Autodesk Inventor part; units mm, degrees
ref_plane "YZ Plane" through (0, 0, 0) normal (1, 0, 0) x (0, 1, 0)
ref_plane "XZ Plane" through (0, 0, 0) normal (0, 1, 0) x (-1, 0, 0)
ref_plane "XY Plane" through (0, 0, 0) normal (0, 0, 1) x (1, 0, 0)
sketch "Sketch1" plane through (0, 0, 0) normal (0, 0, 1) x (1, 0, 0)
  line L0 (-35, 35) -> (35, 35)
  line L1 (35, 35) -> (35, -35)
  line L2 (35, -35) -> (-35, -35)
  line L3 (-35, -35) -> (-35, 35)
  circle A0 centre (0, 0) radius 20
  point P0 (35, 0)
  point P1 (0, 35)
  dimension "d0" = 70
  dimension "d1" = 40
extrude "Extrusion1" add sketch "Sketch1" along normal blind 6
chamfer "Chamfer1" distance 12 angle 45 4 edges at (35, 35, 3) (35, -35, 3) (-35, -35, 3) (-35, 35, 3)
fillet "Fillet1" radius 2 8 edges at (-23, 35, 3) (23, 35, 3) (35, 23, 3) (35, -23, 3) (23, -35, 3) (-23, -35, 3) (-35, -23, 3) (-35, 23, 3)
sketch "Sketch2" plane through (0, 0, 6) normal (0, 0, 1) x (1, 0, 0)
  circle A0 centre (0, 0) radius 32 construction
  point P0 (32, 0)
  dimension "d8" = 64
hole "Hole1" at (32, 0, 6) direction (0, 0, -1) diameter 5.1 end through all
pattern_circular "Circular Pattern1" count 4 over 360 about axis through (0, 0, -10) along (0, 0, 1) of "Hole1"
sketch "Sketch3" plane through (0, 0, 6) normal (0, 0, 1) x (1, 0, 0)
  circle A0 centre (0, 0) radius 23.75 construction
  point P0 (23.75, 0)
  dimension "d19" = 47.5
hole "Hole2" at (23.75, 0, 6) direction (0, 0, -1) diameter 3.2 end through all
pattern_circular "Circular Pattern2" count 4 over 360 about axis through (0, 0, -10) along (0, 0, 1) of "Hole2"
properties part number "plasma-box-spacer-6mm" material "Copper"
Verification items for the finished model (mm, model axes). Give positions to 0.01 mm unless a question says otherwise; leave off trailing zeros. Order: outer loops, then holes, each group sorted by start corner. A loop starts at its lowest first (then second) coordinate and runs counter-clockwise, first axis right, second up. Notation, with made-up numbers: M 29.5,40.25 L 84.5,40.25 A11 cw 84.5,44.25 Z; hole C -12,-17 d7. An arc over 180 degrees is marked long. Use one line per item in the form item = value. Start each with the question number.
Q1. Section check B-B (y = 0). Enter the section's corners in (x, z), then the cut area to 3 significant figures.
Q2. Scan lines: line 1 along Y through (x, z) = (0, 1.7); line 2 along Y through (x, z) = (-2, 2.25); line 3 along Y through (x, z) = (-30.5, 4.65). Record each from-to range of solid material in increasing order. Write a range as [from, to].
Q3. Section check A-A (x = 32). Enter the section's corners in (y, z), then the cut area to 3 significant figures.
Q4. Go/stop test with a flat-tipped pin: pin 1 Ø1.9 at (x, y) = (-23.75, 0) entering from +Z. Record where the tip stops, or that it passes through.
Q5. Section check C-C (z = 4.4). Count the separate pieces of the cut face and the enclosed holes in it, then the cut area to 3 significant figures.
Q6. Mould release check, pull along X, two halves, no side actions. Record for faces 1 (the flat face through (29, 29, 3)), 2 (the flat face through (15, 16, 0)), 3 (the cylindrical face through (-22.164, -0.208, 2.958)): +X half, -X half, draft (parallel to the pull), parting line (faces both ways), or undercut.
Evaluation:
q1.outline = M -35,0 L -34.55,0 L -34.55,6 L -35,6 Z; M -29.45,0 L -25.35,0 L -25.35,6 L -29.45,6 Z; M -22.15,0 L -20,0 L -20,6 L -22.15,6 Z; M 20,0 L 22.15,0 L 22.15,6 L 20,6 Z; M 25.35,0 L 29.45,0 L 29.45,6 L 25.35,6 Z; M 34.55,0 L 35,0 L 35,6 L 34.55,6 Z
q1.area = 80.4 mm2
q2.line_1 = [-35, -34.55], [-29.45, -25.35], [-22.15, -20], [20, 22.15], [25.35, 29.45], [34.55, 35]
q2.line_2 = [-35, -33.58], [-30.42, -19.9], [19.9, 30.42], [33.58, 35]
q2.line_3 = [-27.5, -2.06], [2.06, 27.5]
q3.outline = M -26,0 L -2.55,0 L -2.55,6 L -26,6 Z; M 2.55,0 L 26,0 L 26,6 L 2.55,6 Z
q3.area = 281 mm2
q4.pin_1 = through
q5.separate_pieces = 1
q5.enclosed_holes = 9
q5.area = 3,240 mm2
q6.face_1 = +X half
q6.face_2 = draft
q6.face_3 = undercut
